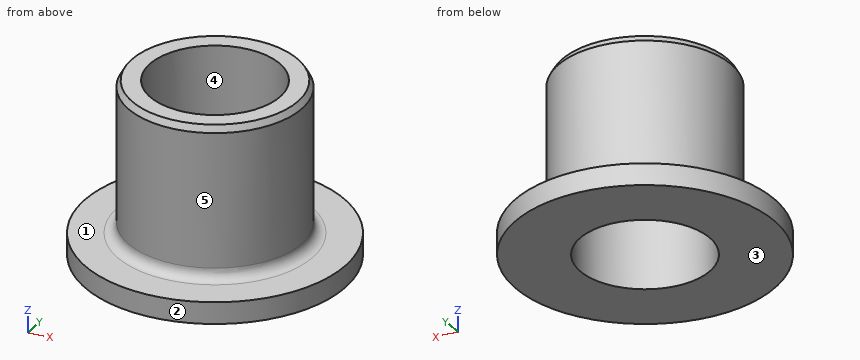
from build123d import *


with BuildPart() as part:
    # Sketch1 → Revolve1 (revolve)
    with BuildSketch(Plane(origin=(0, 0, 0), x_dir=(0, 0, -1), z_dir=(1, 0, 0))):
        with BuildLine():
            Line((0, 6), (-1, 6))
            Line((-1, 6), (-1, 4.5))
            ThreePointArc((-1, 4.5), (-1.146446609, 4.146446609), (-1.5, 4))
            Line((-1.5, 4), (-7.7, 4))
            Line((-7.7, 4), (-8, 3.826794919))
            Line((-8, 3.826794919), (-8, 3))
            Line((-8, 3), (0, 3))
            Line((0, 3), (0, 6))
        make_face()
    revolve(axis=Axis((0, 0, 0), (0, 0, -1)))


solid = part.part
For this review, take the finished solid that the model builds, in its own axes (mm). Face numbers are marked on the shaded views. A direction names the side the tool comes from. Round coordinates to 2 decimals unless told otherwise and drop trailing zeros. Write each loop counter-clockwise with the first axis right and the second up, starting at its lowest first coordinate (ties: lowest second). Pieces come first, ordered by that corner, then holes. Notation, with made-up numbers: (35, 74) - (69, 74) arc R9 ccw to (69, 80) - close; hole circle Ø6 at (65.25, -14). An arc over 180 degrees is marked (long way). Use a Markdown table: item, result.
Q1. Wall thickness on line 1 along X through (y, z) = (0, 4.5); line 2 along X through (y, z) = (-1.5, 2); line 3 along Y through (x, z) = (1.25, 4.5): over which ranges is each line inside the solid? List them lowest first.
Derived:
| item | result |
|---|---|
| line 1 | x = -4 to -3, 3 to 4 |
| line 2 | x = -3.71 to -2.6, 2.6 to 3.71 |
| line 3 | y = -3.8 to -2.73, 2.73 to 3.8 |
Q2. We need section A-A (x = 0). Give the boundary of the cut face in (y, z).
Derived:
| item | result |
|---|---|
| outline | (-6, 0) - (-3, 0) - (-3, 8) - (-3.83, 8) - (-4, 7.7) - (-4, 1.5) arc R0.5 cw to (-4.5, 1) - (-6, 1) - close; (3, 0) - (6, 0) - (6, 1) - (4.5, 1) arc R0.5 cw to (4, 1.5) - (4, 7.7) - (3.83, 8) - (3, 8) - close |
Q3. The part is to be moulded in two halves that separate along Z. For the marked faces 1, 2 and 3, say which applies: pulls with the +Z half, pulls with the -Z half, needs draft (parallel to the pull), parting line crosses it, or undercut.
Derived:
| item | result |
|---|---|
| face 1 | pulls with the +Z half |
| face 2 | needs draft |
| face 3 | pulls with the -Z half |
Q4. Machinability: for the marked faces 4 and 5, which of the approach directions +Z, -Z, +X, -X, +Y, -Y give a long, thin tool a straight path to every point of the face, cutting with its end or side? Answer none if there is none.
Derived:
| item | result |
|---|---|
| face 4 | +Z, -Z |
| face 5 | +Z |
Q5. Clearance check with flat-ended pins moving along their axes: pin 1 (3 mm diameter, centred on x = -4, z = 4.5, fed in from -Y); pin 2 (1 mm diameter, centred on x = 1, z = 5.5, fed in from -Y); pin 3 (1.5 mm diameter, centred on y = 0, z = 7, fed in from +X); pin 4 (3.5 mm diameter, centred on x = 0, y = 0, fed in from -Z). State where each tip first meets the part, or that it passes through.
Derived:
| item | result |
|---|---|
| pin 1 | stops at y = -3.12 |
| pin 2 | stops at y = -3.97 |
| pin 3 | stops at x = 4 |
| pin 4 | passes through |
Q6. We need section C-C (z = 4.75). Give the boundary of the cut face in (x, y), plus the area to 3 significant figures.
Derived:
| item | result |
|---|---|
| outline | circle Ø8 at (0, 0); hole circle Ø6 at (0, 0) |
| area | 22.0 mm2 |
